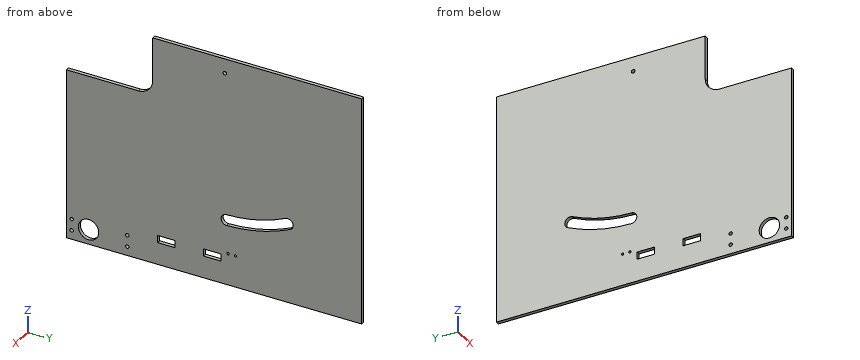
```python
from build123d import *

# Parameters (mm, degrees)
SKETCH1_W           = 200.025
SKETCH1_H           = 260.35
BOSS_EXTRUDE1_DEPTH = 3.175
SKETCH8_R           = 1.55
SKETCH8_R_2         = 1.0499979
CUT_EXTRUDE7_DEPTH  = 4.175
SKETCH9_W           = 50.8
SKETCH9_H           = 76.2
CUT_EXTRUDE8_DEPTH  = 4.175
FILLET1_R           = 12.7
CUT_EXTRUDE9_DEPTH  = 4.175
SKETCH15_W          = 6.35
SKETCH15_H          = 15.24
CUT_EXTRUDE12_DEPTH = 4.175
SKETCH16_R          = 1.5
SKETCH16_R_2        = 9
CUT_EXTRUDE13_DEPTH = 4.175


with BuildPart() as part:
    # Sketch1 → Boss-Extrude1 (new body)
    with BuildSketch(Plane(origin=(0, 0, 0), x_dir=(0, 0, -1), z_dir=(1, 0, 0))):
        Rectangle(SKETCH1_W, SKETCH1_H)
    extrude(amount=BOSS_EXTRUDE1_DEPTH)

    # Sketch8 → Cut-Extrude7 (cut, through all)
    with BuildSketch(Plane.ZY):
        with Locations((87.3125, 9.525)):
            Circle(SKETCH8_R)
        with Locations((-72.3175, 18.9250066)):
            Circle(SKETCH8_R_2)
        with Locations((-72.3175, 12.4249942)):
            Circle(SKETCH8_R_2)
    extrude(amount=-CUT_EXTRUDE7_DEPTH, mode=Mode.SUBTRACT)

    # Sketch9 → Cut-Extrude8 (cut, through all)
    with BuildSketch(Plane.ZY):
        with Locations((74.6125, -92.075)):
            Rectangle(SKETCH9_W, SKETCH9_H)
    extrude(amount=-CUT_EXTRUDE8_DEPTH, mode=Mode.SUBTRACT)

    # Fillet1
    fillet1_edges = [part.edges().sort_by_distance(p)[0] for p in [
        (1.5875, -53.975, 49.2125),
    ]]
    fillet(fillet1_edges, radius=FILLET1_R)

    # Sketch10 → Cut-Extrude9 (cut, through all)
    with BuildSketch(Plane.ZY):
        with BuildLine():
            ThreePointArc((-34.631218673, 67.095364965), (-44.09213985, 39.8142402), (-47.528128749, 11.144346963))
            ThreePointArc((-47.528128749, 11.144346963), (-42.823162504, 6.325000001), (-38.003815542, 11.029966247))
            ThreePointArc((-38.003815542, 11.029966247), (-34.810523806, 37.674794334), (-26.017864022, 63.028948034))
            ThreePointArc((-26.017864022, 63.028948034), (-28.291332832, 69.36883393), (-34.631218673, 67.095364965))
        make_face()
    extrude(amount=-CUT_EXTRUDE9_DEPTH, mode=Mode.SUBTRACT)

    # Sketch15 → Cut-Extrude12 (cut, through all)
    with BuildSketch(Plane(origin=(3.175, 0, 0), x_dir=(0, 0, -1), z_dir=(1, 0, 0))):
        with Locations((77.4925, -1.5450058)):
            Rectangle(SKETCH15_W, SKETCH15_H)
        with Locations((77.4925, -42.1850058)):
            Rectangle(SKETCH15_W, SKETCH15_H)
    extrude(amount=-CUT_EXTRUDE12_DEPTH, mode=Mode.SUBTRACT)

    # Sketch16 → Cut-Extrude13 (cut, through all)
    with BuildSketch(Plane(origin=(3.175, 0, 0), x_dir=(0, 0, -1), z_dir=(1, 0, 0))):
        with Locations((82.075, -125.4125)):
            Circle(SKETCH16_R)
        with Locations((82.075, -76.4125)):
            Circle(SKETCH16_R)
        with Locations((92.075, -125.4125)):
            Circle(SKETCH16_R)
        with Locations((92.075, -76.4125)):
            Circle(SKETCH16_R)
        with Locations((87.075, -110.5624916)):
            Circle(SKETCH16_R_2)
    extrude(amount=-CUT_EXTRUDE13_DEPTH, mode=Mode.SUBTRACT)


solid = part.part
```
The listing builds one solid part. Answer for the finished solid, in the listing's coordinates (mm). Round coordinates to 2 decimals unless told otherwise and drop trailing zeros. Loops run counter-clockwise (first coordinate to the right, second up) from the corner with the lowest first, then second, coordinate; pieces in that order, holes last. Notation, with made-up numbers: (-20, 38.5) - (3, 38.5) arc R30 ccw to (3, 73.5) - close; hole circle Ø10 at (5.5, -38.75). An arc over 180 degrees is marked (long way). Use one line per item in the form item = value. Start each with the question number.
1. Given pin 1 Ø1.6 at (x, y) = (1.5, -91.5) entering from +Z; pin 2 Ø20.5 at (y, z) = (-110.56, -87.08) entering from -X, each flat-ended and moving along its own axis, determine where each tip first touches the part or whether it passes through.
2. Consider line 1 (Z direction, x = 1.3, y = -4); line 2 (Y direction, x = 2.85, z = -87) (3 decimals); line 3 (Y direction, x = 0.75, z = -80.5) (3 decimals). Determine where each line is inside the solid, lowest interval first. Write a range as [from, to].
3. The part is cut by section B-B on y = -86.5. Determine the outline of the cut face in (x, z) (1 decimal).
4. The part is cut by section A-A on x = 0.9. Give the number of separate pieces and of enclosed holes in the cut face, then the cut area to 3 significant figures.
Geometry check:
q1.pin_1 = 49.21
q1.pin_2 = 0
q2.line_1 = [-100.01, -80.67], [-74.32, 100.01]
q2.line_2 = [-130.175, -119.562], [-101.563, 130.175]
q2.line_3 = [-130.175, -116.708], [-104.417, -49.805], [-34.565, -9.165], [6.075, 130.175]
q3.outline = (0, -100) - (3.2, -100) - (3.2, 49.2) - (0, 49.2) - close
q4.separate_pieces = 1
q4.enclosed_holes = 11
q4.area = 47,100 mm^2
